from build123d import *

# Parameters (mm, degrees)
F1_DEPTH = 32
F2_R     = 9.5
F3_DEPTH = 19
F2_R_2   = 19.5
F4_DEPTH = 12
F6_DEPTH = 6
F7_W     = 22
F7_H     = 56
F8_DEPTH = 6


with BuildPart() as f1:
    # F0 (on Right) → F1 (new body, symmetric)
    with BuildSketch(Plane.YZ):
        Polygon((0, 0), (140, 0), (140, 19), (10.9696551146, 19), (-45.9256258422, 117.5455173281), (9.5, 149.5455173281), (0, 166), (-71.8801085141, 124.5), align=None)
    extrude(amount=F1_DEPTH, both=True)

    # F2 (on face) → F3 (cut, through all)
    with BuildSketch(Plane(origin=(0, -71.8801085141, 124.5), x_dir=(1, 0, 0), z_dir=(0, -0.5, 0.8660254038))):
        with BuildLine():
            ThreePointArc((2.022e-07, 83), (22.6274170695, 73.6274169265), (32, 51))
            Line((32, 51), (32, 83))
            Line((32, 83), (2.022e-07, 83))
        make_face()
        with BuildLine():
            ThreePointArc((-32, 51), (-22.6274169265, 73.6274170695), (2.022e-07, 83))
            Line((2.022e-07, 83), (-32, 83))
            Line((-32, 83), (-32, 51))
        make_face()
        with Locations((0, 51)):
            Circle(F2_R)
    extrude(amount=-F3_DEPTH, mode=Mode.SUBTRACT)

    # F2 (on face) → F4 (cut)
    with BuildSketch(Plane(origin=(0, -71.8801085141, 124.5), x_dir=(1, 0, 0), z_dir=(0, -0.5, 0.8660254038))):
        with Locations((0, 51)):
            Circle(F2_R_2)
        with Locations((0, 51)):
            Circle(F2_R, mode=Mode.SUBTRACT)
    extrude(amount=-F4_DEPTH, mode=Mode.SUBTRACT)

    # F5 (on face) → F6 (cut)
    with BuildSketch(Plane(origin=(0, -71.8801085141, 124.5), x_dir=(1, 0, 0), z_dir=(0, -0.5, 0.8660254038))):
        with BuildLine():
            Line((-11, 0), (11, 0))
            Line((11, 0), (11, 20.9500415974))
            ThreePointArc((11, 20.9500415974), (0, 19), (-11, 20.9500415974))
            Line((-11, 20.9500415974), (-11, 0))
        make_face()
        with BuildLine():
            ThreePointArc((-11, 20.9500415974), (0, 19), (11, 20.9500415974))
            Line((11, 20.9500415974), (11, 83))
            Line((11, 83), (-11, 83))
            Line((-11, 83), (-11, 20.9500415974))
        make_face()
    extrude(amount=-F6_DEPTH, mode=Mode.SUBTRACT)

    # F7 (on face) → F8 (cut)
    with BuildSketch(Plane(origin=(0, 0, 0), x_dir=(1, 0, 0), z_dir=(0, -0.8660254038, -0.5))):
        with Locations((0, 109.7602170282)):
            Rectangle(F7_W, F7_H)
    extrude(amount=-F8_DEPTH, mode=Mode.SUBTRACT)


solid = f1.part
The listing builds one solid part. Answer for the finished solid, in the listing's coordinates (mm). A direction names the side the tool comes from. Coordinates: 2 decimals unless noted, no trailing zeros. Order: outer loops, then holes, each group sorted by start corner. A loop starts at its lowest first (then second) coordinate and runs counter-clockwise, first axis right, second up.
Q1. A cutting plane is placed at C-C, the plane z = 81. Write down the section's boundary in (x, y).
Q2. A cutting plane is placed at B-B, the plane y = -56.5. Write down the section's boundary in (x, z).
Q3. Given P1, Ø3, axis at x = 21.5, z = 111, coming from the -Y side; P2, Ø6, axis at x = -13, y = -40.5, coming from the -Z side; P3, Ø4, axis at x = 23.5, y = -7, coming from the +Z side, each flat-ended and moving along its own axis, determine where each tip first touches the part or whether it passes through.
Q4. Consider line 1 (Z direction, x = 1.5, y = 23); line 2 (Z direction, x = 4.5, y = -12.5); line 3 (Z direction, x = -20, y = -11.5). Determine where each line is inside the solid, lowest interval first.
Q5. Which of the six approach directions +Z, -Z, +X, -X, +Y, -Y give full straight-line access (tool end or side, diameter ignored) to faces 1 (the face through (11, -56, 108)), 2 (the face through (0.45, -17.08, 67.58)), 3 (the face through (-8.94, -25.229, 137.578)), 4 (the face through (11, -6, 159))?
Q6. A cutting plane is placed at D-D, the plane x = 23. Write down the section's boundary in (y, z).
Q7. A cutting plane is placed at A-A, the plane x = 4.5. Write down the section's boundary in (y, z).
Q8. For a pull along Y with two mould halves and no side action, classify faces 5 (the face through (4.384, -27.286, 132.405)), 6 (the face through (-11, -6, 159)), 7 (the face through (0.448, -36.443, 63.121)) as pulls with the +Y half, pulls with the -Y half, needs draft (parallel to the pull), parting line crosses it, or undercut.
Answers follow:
1. outline: (-32, -46.77) - (-11, -46.77) - (-11, -39.84) - (11, -39.84) - (11, -46.77) - (32, -46.77) - (32, -24.83) - (-32, -24.83) - close
2. outline: (-32, 97.86) - (-11, 97.86) - (-11, 109.86) - (11, 109.86) - (11, 97.86) - (32, 97.86) - (32, 133.38) - (11, 133.38) - (11, 126.45) - (-11, 126.45) - (-11, 133.38) - (-32, 133.38) - close
3. P1: stops at y = -64.95
3. P2: stops at z = 64.95
3. P3: stops at z = 161.85
4. line 1: z = 0 to 19
4. line 2: z = 21.65 to 59.65, 140.38 to 144.93
4. line 3: z = 19.92 to 57.92, 137.42 to 159.36
5. face 1: -Y
5. face 2: +X, -X, +Y
5. face 3: none
5. face 4: +Z, -Y
6. outline: (-71.88, 124.5) - (0, 0) - (140, 0) - (140, 19) - (10.97, 19) - (-45.93, 117.55) - (1.06, 144.67) - (-8.44, 161.12) - close
7. outline: (-63.68, 122.3) - (-35.68, 73.81) - (-40.88, 70.81) - (0, 0) - (140, 0) - (140, 19) - (10.97, 19) - (-45.93, 117.55) - (-25.46, 129.36) - (-28.96, 135.42) - (-38.14, 130.12) - (-41.14, 135.32) - close; (-14.47, 143.79) - (-10.97, 137.73) - (9.22, 149.39) - (2.72, 160.64) - (-8.28, 154.29) - (-5.28, 149.09) - close
8. face 5: undercut
8. face 6: needs draft
8. face 7: pulls with the -Y half
